Read the model definition and answer for the solid it produces. Units are mm, in the model's axes. Face numbers are marked on the shaded views. A direction names the side the tool comes from. Coordinates: 2 decimals unless noted, no trailing zeros. Order: outer loops, then holes, each group sorted by start corner. A loop starts at its lowest first (then second) coordinate and runs counter-clockwise, first axis right, second up. Notation, with made-up numbers: M 88.5,32 L 138.5,32 A21 cw 138.5,42 Z; hole C -22,-21 d8. An arc over 180 degrees is marked long. Use a Markdown table: item, result. Add a question column.
1) Find section A-A on y = 0. Write down the section's boundary in (x, z), plus the area to 3 significant figures.
2) The mould has two halves that part along X. Classify the marked faces 3, 4, 5 and 6: released by +X, released by -X, zero draft, split by the parting line, or undercut.
3) Find section B-B on x = 3. Write down the section's boundary in (y, z).
4) Find the intervals of material crossed by probe 1 along Y at (x, z) = (3, 1.5), in increasing order. Write a range as [from, to].
5) Find section D-D on y = 2.75. Write down the section's boundary in (x, z).
6) Find section C-C on z = -1.25. Write down the section's boundary in (x, y), plus the area to 3 significant figures.
7) Each of these flat-tipped pins is pushed along its axis until it touches: pin 1 Ø5 at (x, y) = (-2, 3) entering from -Z; pin 2 Ø5 at (y, z) = (0, 0) entering from +X. Where does it stop, or does it pass through?
8) For the marked faces 1 and 2, determine the directions among +Z, -Z, +X, -X, +Y, -Y from which every point of the face is accessible in a straight line to the end or side of a thin tool.
from build123d import *

# Parameters (mm, degrees)
F0_W     = 10
F0_H     = 10
F1_DEPTH = 5
F2_T     = -1
F4_D     = 8
F5_D     = 8


with BuildPart() as f1:
    # F0 (on Front) → F1 (new body, symmetric)
    with BuildSketch(Plane.XZ):
        Rectangle(F0_W, F0_H)
    extrude(amount=F1_DEPTH, both=True)

    # F2
    f2_openings = [f1.faces().sort_by_distance(p)[0] for p in [
        (0, 0, 5),
        (0, 0, -5),
    ]]
    offset(amount=F2_T, openings=f2_openings)

    # F4 (through all)
    with Locations(Plane.YZ):
        with Locations((0, 0)):
            Hole(F4_D / 2)

    # F5 (through all)
    with Locations(Plane(origin=(0, 0, 0), x_dir=(0, 1, 0), z_dir=(-1, 0, 0))):
        with Locations((0, 0)):
            Hole(F5_D / 2)


solid = f1.part
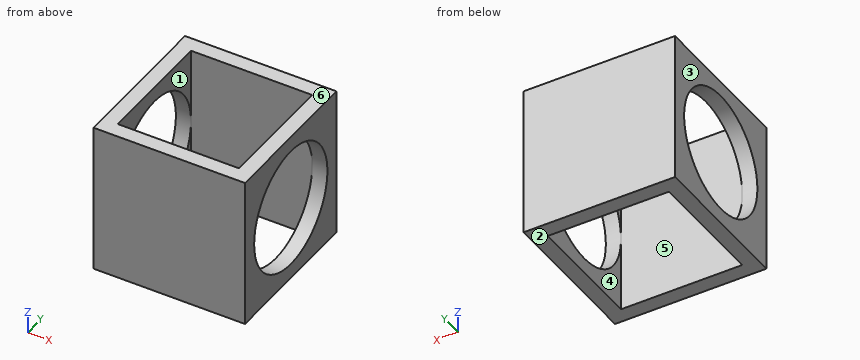
Check result:
| question | item | result |
|---|---|---|
| 1 | outline | M -5,-5 L -4,-5 L -4,-4 L -5,-4 Z; M -5,4 L -4,4 L -4,5 L -5,5 Z; M 4,-5 L 5,-5 L 5,-4 L 4,-4 Z; M 4,4 L 5,4 L 5,5 L 4,5 Z |
| 1 | area | 4.00 mm2 |
| 2 | face 3 | released by -X |
| 2 | face 4 | undercut |
| 2 | face 5 | undercut |
| 2 | face 6 | zero draft |
| 3 | outline | M -5,-5 L -4,-5 L -4,5 L -5,5 Z; M 4,-5 L 5,-5 L 5,5 L 4,5 Z |
| 4 | probe 1 | y = [-5, -4], [4, 5] |
| 5 | outline | M -5,-5 L -4,-5 L -4,-2.9 L -5,-2.9 Z; M -5,2.9 L -4,2.9 L -4,5 L -5,5 Z; M 4,-5 L 5,-5 L 5,-2.9 L 4,-2.9 Z; M 4,2.9 L 5,2.9 L 5,5 L 4,5 Z |
| 6 | outline | M -5,-5 L 5,-5 L 5,-3.8 L 4,-3.8 L 4,-4 L -4,-4 L -4,-3.8 L -5,-3.8 Z; M -5,3.8 L -4,3.8 L -4,4 L 4,4 L 4,3.8 L 5,3.8 L 5,5 L -5,5 Z |
| 6 | area | 20.8 mm2 |
| 7 | pin 1 | stops at z = -5 |
| 7 | pin 2 | passes through |
| 8 | face 1 | +Z, -Z |
| 8 | face 2 | -Z, +X, -X, +Y, -Y |
